Could you check a few things on this drawing? It's one solid part, dimensions in mm from its lowest x, y, z. A direction names the side the tool comes from. Coordinates: 2 decimals unless noted, no trailing zeros. Loops run counter-clockwise (first coordinate to the right, second up) from the corner with the lowest first, then second, coordinate; pieces in that order, holes last. Notation, with made-up numbers: (-33.5, 82) -> (17.5, 82) arc R25 cw to (17.5, 110) -> close; hole circle Ø9 at (36, -6.75). An arc over 180 degrees is marked (long way). One line per question, with ' | ' between items.
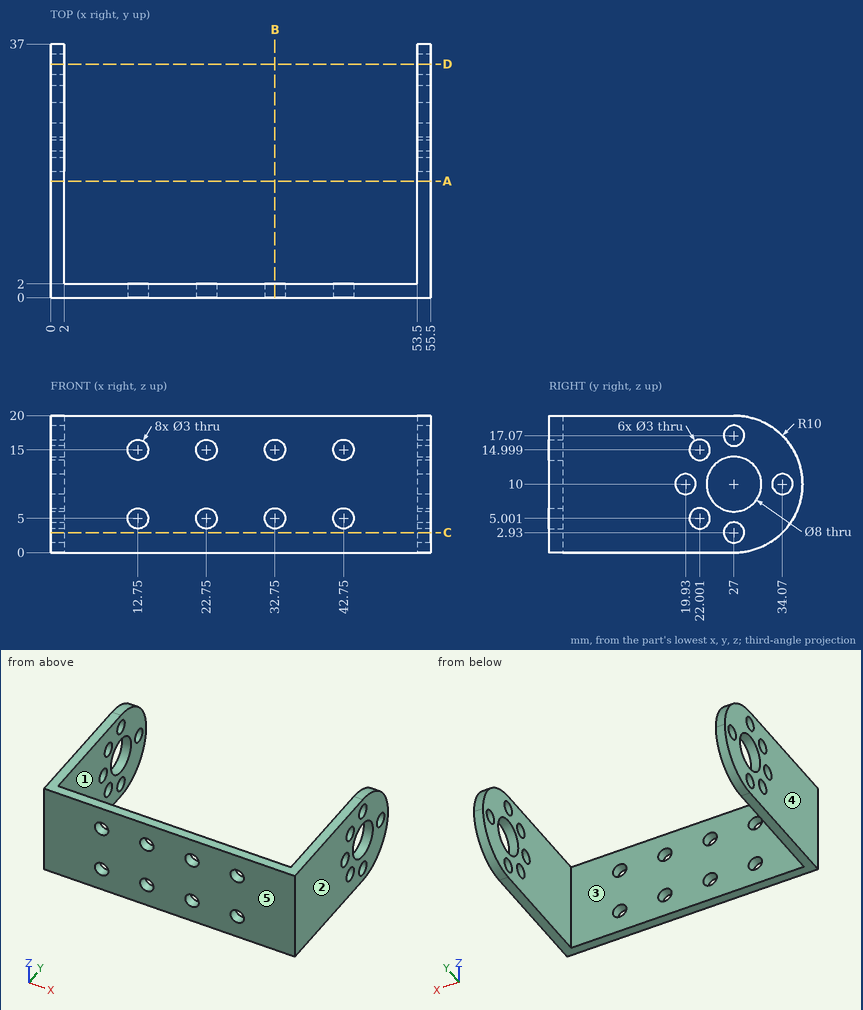
1) On a 3-axis mill with a long thin cutter (end or side, diameter ignored), from which of +Z, -Z, +X, -X, +Y, -Y can I reach the whole of each face in a straight line? I mean the marked faces 1 and 2. Say none if no direction works.
Data:
face 1: +Z, -Z, +Y | face 2: +Z, -Z, +X, +Y, -Y
2) We'd pull the mould along X, two halves only. Please class the marked faces 3, 4 and 5: pulls with the +X half, pulls with the -X half, needs draft (parallel to the pull), parting line crosses it, or undercut.
Data:
face 3: undercut | face 4: pulls with the -X half | face 5: needs draft
3) I need wall thicknesses on line 1 along X through (y, z) = (0.7, 5); line 2 along X through (y, z) = (33.5, 16.5); line 3 along Y through (x, z) = (26, 11.25). Which ranges of each line are inside material? Lowest first, please. Write a range as from..to.
Data:
line 1: 0..11.25, 14.25..21.25, 24.25..31.25, 34.25..41.25, 44.25..55.5 | line 2: 0..2, 53.5..55.5 | line 3: 0..2
4) If we section it at B-B on x = 32.75: Please give me the cut outline in (y, z), and give its area (3 significant figures).
Data:
outline: (0, 0) -> (2, 0) -> (2, 3.5) -> (0, 3.5) -> close; (0, 6.5) -> (2, 6.5) -> (2, 13.5) -> (0, 13.5) -> close; (0, 16.5) -> (2, 16.5) -> (2, 20) -> (0, 20) -> close | area: 28.0 mm²
5) If we section it at A-A on y = 17: Please give me the cut outline in (x, z).
Data:
outline: (0, 0) -> (2, 0) -> (2, 20) -> (0, 20) -> close; (53.5, 0) -> (55.5, 0) -> (55.5, 20) -> (53.5, 20) -> close
6) I'm going to push a flat-ended pin straight in: pin 1 Ø5 at (x, z) = (42.75, 15) entering from +Y. Where does the tip first touch, or does it pass through?
Data:
pin 1: y = 2
7) If we section it at C-C on z = 2.93: Please give me the cut outline in (x, y), and give its area (3 significant figures).
Data:
outline: (0, 0) -> (55.5, 0) -> (55.5, 25.5) -> (53.5, 25.5) -> (53.5, 2) -> (2, 2) -> (2, 25.5) -> (0, 25.5) -> close; (0, 28.5) -> (2, 28.5) -> (2, 34.07) -> (0, 34.07) -> close; (53.5, 28.5) -> (55.5, 28.5) -> (55.5, 34.07) -> (53.5, 34.07) -> close | area: 227 mm²
8) If we section it at D-D on y = 34.07: Please give me the cut outline in (x, z).
Data:
outline: (0, 2.93) -> (2, 2.93) -> (2, 8.5) -> (0, 8.5) -> close; (0, 11.5) -> (2, 11.5) -> (2, 17.07) -> (0, 17.07) -> close; (53.5, 2.93) -> (55.5, 2.93) -> (55.5, 8.5) -> (53.5, 8.5) -> close; (53.5, 11.5) -> (55.5, 11.5) -> (55.5, 17.07) -> (53.5, 17.07) -> close
